Design review of the part built by this model. Coordinates are the model's own, in mm. A direction names the side the tool comes from. Coordinates: 2 decimals unless noted, no trailing zeros. Loops run counter-clockwise (first coordinate to the right, second up) from the corner with the lowest first, then second, coordinate; pieces in that order, holes last.
Q1. For P1, Ø3, axis at y = 18, z = 39.5, coming from the -X side; P2, Ø1.5, axis at y = 9, z = 29, coming from the +X side; P3, Ø13, axis at x = 34, y = -15, coming from the +Z side, all flat-tipped, find the tip position at first contact; note any pin that passes through.
Q2. Machinability: for faces 1 (the face through (8.96, -8.72, 87.32)), 2 (the face through (-25, 0, 4)), 3 (the face through (-8.72, -8.96, 87.32)), 4 (the face through (-8.96, 8.72, 87.32)), 5 (the face through (-39, 19, 10)), which of the approach directions +Z, -Z, +X, -X, +Y, -Y give a long, thin tool a straight path to every point of the face, cutting with its end or side? Answer none if there is none.
Q3. Wall thickness on probe 1 along Y at (x, z) = (35, 4); probe 2 along Y at (x, z) = (35, 12); probe 3 along Z at (x, y) = (-29.5, -5.5): over which ranges is each line inside the solid? List them lowest first.
Q4. Draft analysis for pull direction X (two halves, no side actions). For faces 6 (the face through (-35, 0, 0)), 7 (the face through (10.382, 19.961, 45.594)), 8 (the face through (30, 15, 5)), state which applies: released by +X, released by -X, zero draft, split by the parting line, or undercut.
Q5. Add section B-B on z = 45. Give the boundary of the cut face in (x, y), and give its area (3 significant figures).
Q6. Add section A-A on z = 92. Give the boundary of the cut face in (x, y), and give its area (3 significant figures).
Autodesk Inventor part; units mm, degrees
ref_plane "YZ Plane" through (0, 0, 0) normal (1, 0, 0) x (0, 1, 0)
ref_plane "XZ Plane" through (0, 0, 0) normal (0, 1, 0) x (-1, 0, 0)
ref_plane "XY Plane" through (0, 0, 0) normal (0, 0, 1) x (1, 0, 0)
sketch "Sketch1" plane through (0, 0, 0) normal (0, 0, 1) x (1, 0, 0)
  line L0 (-65.8995, 0) -> (65.8995, 0)
  line L1 (0, -37.8995) -> (0, 37.8995)
  line L2 (-45, 0) -> (-45, 15)
  line L3 (-35, 25) -> (0, 25)
  arc A0 (-35, 25) -> (-45, 15) centre (-35, 15) ccw
  circle A1 centre (-35, 15) radius 5
  circle A2 centre (-35, 15) radius 6
  circle A3 centre (-35, -15) radius 6
  circle A4 centre (35, 15) radius 6
  circle A5 centre (35, -15) radius 6
  circle A6 centre (-35, -15) radius 5
  circle A7 centre (35, 15) radius 5
  circle A8 centre (35, -15) radius 5
  line L4 (-45, 0) -> (-45, -15)
  line L5 (-35, -25) -> (0, -25)
  arc A9 (-45, -15) -> (-35, -25) centre (-35, -15) ccw
  line L6 (45, 0) -> (45, 15)
  line L7 (35, 25) -> (0, 25)
  arc A10 (45, 15) -> (35, 25) centre (35, 15) ccw
  line L8 (35, -25) -> (0, -25)
  arc A11 (35, -25) -> (45, -15) centre (35, -15) ccw
  line L9 (45, 0) -> (45, -15)
  point P0 (0, 0)
  point P1 (-45, 25)
  point P2 (-45, -25)
  point P3 (45, 25)
  dimension "d3" = 50
  dimension "d4" = 90
  dimension "d6" = 10
  dimension "d10" = 5
  dimension "d14" = 6
extrude "Extrusion1" add sketch "Sketch1" along normal blind 15 contours L2 A0 L3 L1 L0 | L0 L1 L5 A9 L4 | L1 L7 A10 L6 L0 | L0 L9 A11 L8 L1
extrude "Extrusion2" add sketch "Sketch1" along normal blind 10 contours A2 | A3 | A4 | A5
sketch "Sketch2" plane through (-35, -25, 0) normal (0, -1, 0) x (1, 0, 0)
  line L0 (0, 0) -> (70, 0)
  line L1 (35, -3) -> (35, 18)
  line L2 (10, 7) -> (10, 0)
  line L3 (60, 7) -> (60, 0)
  line L4 (10, 7) -> (60, 7)
  line L5 (10, 0) -> (60, 0)
  point P0 (35, 0)
  dimension "d20" = 7
  dimension "d21" = 50
extrude "Extrusion3" cut sketch "Sketch2" against normal blind 50
sketch "Sketch3" plane through (0, 0, 15) normal (0, 0, 1) x (1, 0, 0)
  circle A0 centre (0, 0) radius 22.5
  dimension "d24" = 22.5
extrude "Extrusion4" add sketch "Sketch3" along normal blind 60
sketch "Sketch4" plane through (0, 0, 75) normal (0, 0, 1) x (1, 0, 0)
  circle A0 centre (0, 0) radius 22.5
  line L0 (-17.6777, 0) -> (0, 17.6777)
  line L1 (0, 17.6777) -> (17.6777, 0)
  line L2 (17.6777, 0) -> (0, -17.6777)
  line L3 (0, -17.6777) -> (-17.6777, 0)
  dimension "d30" = 25
  dimension "d31" = 25
  dimension "d32" = 25
  dimension "d33" = 25
extrude "Extrusion5" add sketch "Sketch4" along normal blind 25 contours L0 L1 L2 L3
fillet "Fillet1" radius 2 1 edges at (-22.5, 0, 15)
hole "Hole1" at (0, 0, 100) direction (0, 0, -1) diameter 16 depth 20
hole "Hole2" at (0, 0, 80) direction (0, 0, -1) diameter 12 depth 10 tip angle 118
sketch "Sketch5" plane through (0, 0, 0) normal (1, 0, 0) x (0, 1, 0)
  line L0 (0, -20) -> (0, 120)
  line L1 (-25, 7) -> (25, 7)
  line L2 (-35, 0) -> (35, 0)
  line L3 (-15, 8.1453) -> (-15, 51.4254)
  line L4 (-15, 15) -> (15, 15)
  arc A0 (0, 66.4254) -> (-15, 51.4254) centre (0, 51.4254) ccw
  line L5 (0, 66.4254) -> (0, 7)
  line L6 (0, 7) -> (-15, 7)
  line L7 (0, 66.4254) -> (0, 7)
  point P0 (0, 0)
  point P1 (0, 15)
  point P2 (0, 15)
  point P3 (0, 15)
  dimension "d57" = 15
properties part number "Piesa 2 3D"
Entries:
1. P1: stops at x = -15.3
1. P2: stops at x = 20.93
1. P3: stops at z = 15
2. face 1: +Z, +X, -Y
2. face 2: -Z, +Y, -Y
2. face 3: +Z, -X, -Y
2. face 4: +Z, -X, +Y
2. face 5: +Z
3. probe 1: y = -25 to -20, -10 to 10, 20 to 25
3. probe 2: y = -25 to -21, -9 to 9, 21 to 25
3. probe 3: z = 0 to 15
4. face 6: zero draft
4. face 7: split by the parting line
4. face 8: undercut
5. outline: circle Ø45 at (0, 0)
5. area: 1,590 mm2
6. outline: (-17.68, 0) - (0, -17.68) - (17.68, 0) - (0, 17.68) - close; hole circle Ø16 at (0, 0)
6. area: 424 mm2
